from build123d import *

# Parameters (mm, degrees)
F0_W     = 150
F0_H     = 25
F1_DEPTH = 25
F2_W     = 125
F2_H     = 11
F3_DEPTH = 25.001
F5_D     = 4.2


with BuildPart() as f1:
    # F0 (on Front) → F1 (new body)
    with BuildSketch(Plane.XZ):
        with Locations((75, 12.5)):
            Rectangle(F0_W, F0_H)
    extrude(amount=-F1_DEPTH)

    # F2 (on face) → F3 (cut, through all)
    with BuildSketch(Plane.XY.offset(25)):
        with Locations((87.5, 12.5)):
            Rectangle(F2_W, F2_H)
    extrude(amount=-F3_DEPTH, mode=Mode.SUBTRACT)

    # F5 (through all)
    with Locations(Plane(origin=(0, 0, 0), x_dir=(0, -1, 0), z_dir=(-1, 0, 0))):
        with Locations((-12.5, 12.5)):
            Hole(F5_D / 2)


solid = f1.part
Design review of the part built by this model. Coordinates are the model's own, in mm. A direction names the side the tool comes from. Coordinates: 2 decimals unless noted, no trailing zeros. Loops run counter-clockwise (first coordinate to the right, second up) from the corner with the lowest first, then second, coordinate; pieces in that order, holes last. Notation, with made-up numbers: (58, -36.5) -> (70, -36.5) arc R4 ccw to (70, -30.5) -> close; hole circle Ø3 at (66, 12.5). An arc over 180 degrees is marked (long way). Use a Markdown table: item, result. Add a question column.
Item 1: Clearance check with flat-ended pins moving along their axes: P1, Ø3, axis at y = 13, z = 11.5, coming from the +X side; P2, Ø1, axis at x = 59.5, y = 18.5, coming from the -Z side. State where each tip first meets the part, or that it passes through.
Item 2: We need section C-C, the plane z = 12.5. Write out the cut boundary in (x, y), and give its area (3 significant figures).
Item 3: We need section D-D, the plane x = 22.5. Write out the cut boundary in (y, z), and give its area (3 significant figures).
Item 4: The part is to be moulded in two halves that separate along Y. For faces 1 (the flat face through (74, 25, 13)), 2 (the flat face through (0, 12, 10)), 3 (the flat face through (87, 7, 13)), say which applies: +Y half, -Y half, draft (parallel to the pull), parting line (faces both ways), or undercut.
Item 5: Wall thickness on L1, parallel to Y at x = 136.5, z = 11.5; L2, parallel to Z at x = 16, y = 12.5; L3, parallel to X at y = 9.75, z = 9.5: over which ranges is each line inside the solid? List them lowest first. Write a range as from..to.
Item 6: Machinability: for faces 4 (the flat face through (87, 18, 13)), 5 (the flat face through (57.3, 6.8, 0)), which of the approach directions +Z, -Z, +X, -X, +Y, -Y give a long, thin tool a straight path to every point of the face, cutting with its end or side? Answer none if there is none.
Item 7: We need section B-B, the plane y = 12.5. Write out the cut boundary in (x, z).
Item 8: We need section A-A, the plane x = 96. Write out the cut boundary in (y, z), and give its area (3 significant figures).
Numbers:
| question | item | result |
|---|---|---|
| 1 | P1 | stops at x = 25 |
| 1 | P2 | stops at z = 0 |
| 2 | outline | (0, 0) -> (150, 0) -> (150, 7) -> (25, 7) -> (25, 10.4) -> (0, 10.4) -> close; (0, 14.6) -> (25, 14.6) -> (25, 18) -> (150, 18) -> (150, 25) -> (0, 25) -> close |
| 2 | area | 2,270 mm^2 |
| 3 | outline | (0, 0) -> (25, 0) -> (25, 25) -> (0, 25) -> close; hole circle Ø4.2 at (12.5, 12.5) |
| 3 | area | 611 mm^2 |
| 4 | face 1 | +Y half |
| 4 | face 2 | draft |
| 4 | face 3 | undercut |
| 5 | L1 | y = 0..7, 18..25 |
| 5 | L2 | z = 0..10.4, 14.6..25 |
| 5 | L3 | x = 0..25 |
| 6 | face 4 | +Z, -Z, +X |
| 6 | face 5 | -Z, +X, -X, +Y, -Y |
| 7 | outline | (0, 0) -> (25, 0) -> (25, 10.4) -> (0, 10.4) -> close; (0, 14.6) -> (25, 14.6) -> (25, 25) -> (0, 25) -> close |
| 8 | outline | (0, 0) -> (7, 0) -> (7, 25) -> (0, 25) -> close; (18, 0) -> (25, 0) -> (25, 25) -> (18, 25) -> close |
| 8 | area | 350 mm^2 |
